Could you check a few things on this model? Use its own coordinates, in mm. Round coordinates to 2 decimals unless told otherwise and drop trailing zeros. Loops run counter-clockwise (first coordinate to the right, second up) from the corner with the lowest first, then second, coordinate; pieces in that order, holes last. Notation, with made-up numbers: (-26.75, 55) -> (20.25, 55) arc R23 cw to (20.25, 82) -> close; hole circle Ø1 at (66.25, 44). An arc over 180 degrees is marked (long way). Use CSV: the item, a comma, the result in double quotes. Start each with the question number.
Autodesk Inventor part; units mm, degrees
ref_plane "YZ Plane" through (0, 0, 0) normal (1, 0, 0) x (0, 1, 0)
ref_plane "XZ Plane" through (0, 0, 0) normal (0, 1, 0) x (-1, 0, 0)
ref_plane "XY Plane" through (0, 0, 0) normal (0, 0, 1) x (1, 0, 0)
sketch "Sketch1" plane through (0, 0, 0) normal (0, 0, 1) x (1, 0, 0)
  circle A0 centre (-45.2437, 35.97) radius 1.27
  circle A1 centre (-45.2437, 35.97) radius 1.27
  circle A2 centre (10.6363, 0) radius 3.175
  line L0 (-76.9938, -50.8) -> (-76.9938, 50.8)
  line L1 (76.9938, -50.8) -> (-76.9938, -50.8)
  line L2 (76.9938, 50.8) -> (76.9938, -50.8)
  line L3 (-76.9938, 50.8) -> (76.9938, 50.8)
  line L4 (-70.6437, 50.8) -> (29.0843, 50.8)
  line L5 (35.4343, 44.45) -> (35.4343, -44.45)
  line L6 (29.0843, -50.8) -> (-70.6437, -50.8)
  line L7 (-76.9937, -44.45) -> (-76.9938, 44.45)
  arc A3 (-70.6437, 50.8) -> (-76.9938, 44.45) centre (-70.6437, 44.45) ccw
  arc A4 (29.0843, -50.8) -> (35.4343, -44.45) centre (29.0843, -44.45) ccw
  arc A5 (35.4343, 44.45) -> (29.0843, 50.8) centre (29.0843, 44.45) ccw
  arc A6 (-76.9937, -44.45) -> (-70.6437, -50.8) centre (-70.6437, -44.45) ccw
  circle A7 centre (-7.7961, 43.4062) radius 3.175
  circle A8 centre (-32.0501, 9.7076) radius 3.175
  point P0 (0, 0)
  point P1 (35.4343, -50.8)
  dimension "d0" = 6.35
extrude "Extrusion1" add sketch "Sketch1" along normal blind 6.35 contours L0 A3 L3 A5 L5 A4 L1 A6 | A7 | A8
sketch "Sketch2" plane through (0, 0, 6.35) normal (0, 0, 1) x (1, 0, 0)
  circle A0 centre (-45.2437, 35.97) radius 1.27
  circle A1 centre (-7.7961, 43.4062) radius 3.175
  circle A2 centre (-32.0501, 9.7076) radius 3.175
  circle A3 centre (-45.2437, 35.97) radius 3.175
  point P0 (0, 0)
extrude "Extrusion2" cut sketch "Sketch2" against normal through all
sketch "Sketch3" plane through (0, 0, 6.35) normal (0, 0, 1) x (1, 0, 0)
  arc A0 (-12.0087, -29.8172) -> (-8.9086, -33.4326) centre (-11.0366, -32.1205) ccw
  circle A1 centre (-11.0366, -32.1205) radius 2.5
  point P0 (0, 0)
extrude "Extrusion3" cut sketch "Sketch3" against normal through all
properties part number "projectorMountingPlate"
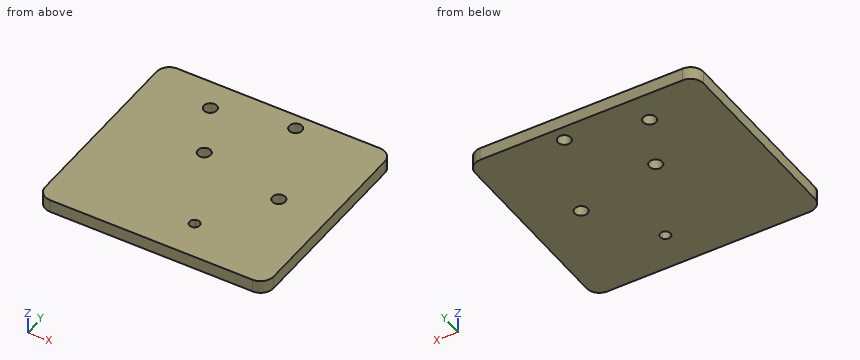
1. Suppose I cut it at C-C (z = 1.25). State how many separate pieces and enclosed holes the cut face has, then the cut area to 3 significant figures.
2. Will this pin go through, and if not, where does the flat tip stop? pin 1 (4 mm diameter, centred on x = -45.24, y = 35.97, fed in from +Z).
3. Suppose I cut it at B-B (x = 10.5). List the corners of the cut face in (y, z) for me.
4. Suppose I cut it at A-A (y = 35.97). List the corners of the cut face in (x, z) for me, then the cut area to 3 significant figures.
5. If I drill on L1, parallel to Y at x = -45, z = 3.25; L2, parallel to X at y = 1, z = 1.75; L3, parallel to Y at x = -5.5, z = 2.75, over which ranges is the centre line in solid material (lowest first)?
Geometry check:
1,separate pieces,"1"
1,enclosed holes,"5"
1,area,"11,200 mm²"
2,pin 1,"passes through"
3,outline,"(-50.8, 0) -> (-3.17, 0) -> (-3.17, 6.35) -> (-50.8, 6.35) -> close; (3.17, 0) -> (50.8, 0) -> (50.8, 6.35) -> (3.17, 6.35) -> close"
4,outline,"(-76.99, 0) -> (-48.42, 0) -> (-48.42, 6.35) -> (-76.99, 6.35) -> close; (-42.07, 0) -> (35.43, 0) -> (35.43, 6.35) -> (-42.07, 6.35) -> close"
4,area,"674 mm²"
5,L1,"y = -50.8 to 32.8, 39.14 to 50.8"
5,L2,"x = -76.99 to 7.62, 13.65 to 35.43"
5,L3,"y = -50.8 to 41.21, 45.6 to 50.8"
